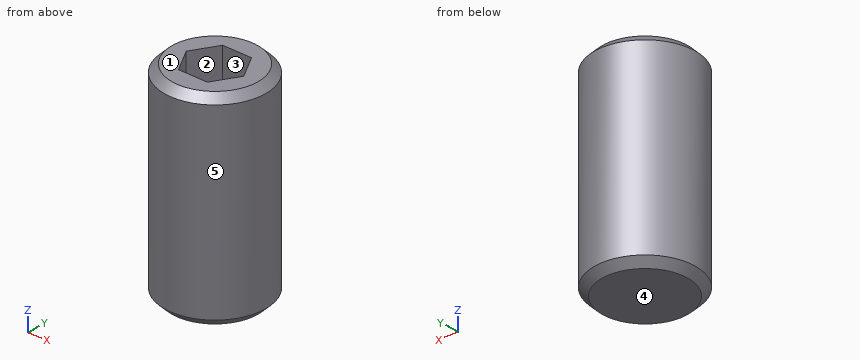
Solid Edge part; units mm, degrees
sketch "Sketch1" plane through (0, 0, 0) normal (0, 0, 1) x (1, 0, 0)
  circle A0 centre (0, 0) radius 3
extrude "Protrusion1" add sketch "Sketch1" along normal mid plane 12
chamfer "Chamfer1" distance 0.45 angle 45 2 edges at (-3, 0, -6) (-3, 0, 6)
sketch "Sketch2" plane through (0, 0, 6) normal (0, 0, 1) x (1, 0, 0)
  line L0 (-0.866, 1.5) -> (0.866, 1.5)
  line L1 (1.7321, 0) -> (0.866, 1.5)
  line L2 (0.866, -1.5) -> (1.7321, 0)
  line L3 (-0.866, -1.5) -> (0.866, -1.5)
  line L4 (-1.7321, 0) -> (-0.866, -1.5)
  line L5 (-0.866, 1.5) -> (-1.7321, 0)
extrude "Cutout1" cut sketch "Sketch2" against normal blind 6
properties part number "185797" material "Stainless Steel, 304"
The model under review builds one solid part; all positions refer to its coordinate system, in mm. Face numbers are marked on the shaded views. A direction names the side the tool comes from. Coordinates: 2 decimals unless noted, no trailing zeros. Write each loop counter-clockwise with the first axis right and the second up, starting at its lowest first coordinate (ties: lowest second). Pieces come first, ordered by that corner, then holes. Notation, with made-up numbers: (37.25, 4) - (90.25, 4) arc R22 ccw to (90.25, 27) - close; hole circle Ø2 at (-24.75, -12). An arc over 180 degrees is marked (long way). Answer in a Markdown table with one row per item. Add a question column.
Q1. For the marked faces 1 and 2, list the 3-axis set-ups (+Z, -Z, +X, -X, +Y, -Y) from which the entire face can be reached by the end or side of a thin tool; tool diameter is ignored.
Q2. Consider section A-A on z = 1.5. Give the boundary of the cut face in (x, y), then the cut area to 3 significant figures.
Q3. Consider section C-C on z = -0.75. Give the boundary of the cut face in (x, y).
Q4. Clearance check with flat-ended pins moving along their axes: pin 1 (1.5 mm diameter, centred on y = -2, z = 0.5, fed in from +X); pin 2 (1.5 mm diameter, centred on x = 1, z = -1.5, fed in from +Y); pin 3 (1.5 mm diameter, centred on x = 0, y = -0.5, fed in from +Z). State where each tip first meets the part, or that it passes through.
Q5. Draft analysis for pull direction Y (two halves, no side actions). For the marked faces 3, 4 and 5, state which applies: +Y half, -Y half, draft (parallel to the pull), parting line (faces both ways), or undercut.
Q6. To check wall thickness, follow line 1 along Y through (x, z) = (0, 4.25); line 2 along Z through (x, y) = (0.4, -0.7); line 3 along X through (y, z) = (0.8, 5.5). State the ranges of each line that lie inside material, in increasing order. Write a range as from..to.
Q7. Consider section B-B on x = 0. Give the boundary of the cut face in (y, z), then the cut area to 3 significant figures.
Answers below:
| question | item | result |
|---|---|---|
| 1 | face 1 | +Z, +X, -X, +Y, -Y |
| 1 | face 2 | +Z |
| 2 | outline | circle Ø6 at (0, 0); hole (-1.73, 0) - (-0.87, -1.5) - (0.87, -1.5) - (1.73, 0) - (0.87, 1.5) - (-0.87, 1.5) - close |
| 2 | area | 20.5 mm² |
| 3 | outline | circle Ø6 at (0, 0) |
| 4 | pin 1 | x = 2.73 |
| 4 | pin 2 | y = 2.99 |
| 4 | pin 3 | z = 0 |
| 5 | face 3 | undercut |
| 5 | face 4 | draft |
| 5 | face 5 | parting line |
| 6 | line 1 | -3..-1.5, 1.5..3 |
| 6 | line 2 | -6..0 |
| 6 | line 3 | -2.89..-1.27, 1.27..2.89 |
| 7 | outline | (-3, -5.55) - (-2.55, -6) - (2.55, -6) - (3, -5.55) - (3, 5.55) - (2.55, 6) - (1.5, 6) - (1.5, 0) - (-1.5, 0) - (-1.5, 6) - (-2.55, 6) - (-3, 5.55) - close |
| 7 | area | 53.6 mm² |
